from build123d import *

# Parameters (mm, degrees)
BOSS_EXTRUDE1_DEPTH                             = 76.2
BOSS_EXTRUDE1_DEPTH_BACK                        = 76.2
SKETCH3_W                                       = 76.2
SKETCH3_H                                       = 6.35
SKETCH11_R                                      = 13.97
CUT_EXTRUDE1_DEPTH                              = 86.430512699
CSK_FOR_M4_FLAT_HEAD_MACHINE_SCREW1_D           = 4.5
CSK_FOR_M4_FLAT_HEAD_MACHINE_SCREW1_CSINK_D     = 9.4
CSK_FOR_M4_FLAT_HEAD_MACHINE_SCREW1_CSINK_ANGLE = 90
SKETCH20_W                                      = 76.2
SKETCH20_H                                      = 76.2
CUT_EXTRUDE2_DEPTH                              = 86.430512699
M3X0_5_TAPPED_HOLE3_D                           = 2.5
M3X0_5_TAPPED_HOLE3_DEPTH                       = 11.948924226
M3X0_5_TAPPED_HOLE3_TIP                         = 0.751075774


with BuildPart() as part:
    # Sketch3 → Boss-Extrude1 (new, two sides: drawn at the far end of the back side and taken through both)
    with BuildSketch(Plane.XY.offset(-BOSS_EXTRUDE1_DEPTH_BACK)):
        Rectangle(SKETCH3_W, SKETCH3_H)
    extrude(amount=BOSS_EXTRUDE1_DEPTH + BOSS_EXTRUDE1_DEPTH_BACK)

    # Sketch11 → Cut-Extrude1 (cut, through all)
    with BuildSketch(Plane.XZ.offset(3.175)):
        with Locations(Location((-0.450951641, 31.810066373, 0), (0, 0, 270))):
            Circle(SKETCH11_R)
    extrude(amount=-CUT_EXTRUDE1_DEPTH, mode=Mode.SUBTRACT)

    # CSK for M4 Flat Head Machine Screw1 (through all)
    with Locations(Plane(origin=(0, -3.175, 0), x_dir=(-1, 0, 0), z_dir=(0, -1, 0))):
        with Locations((11.200951641, -13.190520192), (-21.049048359, -31.810066373), (11.200951641, -50.429612554)):
            CounterSinkHole(CSK_FOR_M4_FLAT_HEAD_MACHINE_SCREW1_D / 2, CSK_FOR_M4_FLAT_HEAD_MACHINE_SCREW1_CSINK_D / 2, counter_sink_angle=CSK_FOR_M4_FLAT_HEAD_MACHINE_SCREW1_CSINK_ANGLE)

    # Sketch20 → Cut-Extrude2 (cut, through all)
    with BuildSketch(Plane.XZ.offset(3.175)):
        with Locations((0, -38.1)):
            Rectangle(SKETCH20_W, SKETCH20_H)
    extrude(amount=-CUT_EXTRUDE2_DEPTH, mode=Mode.SUBTRACT)

    # M3x0.5 Tapped Hole3
    with Locations(Plane.XY.offset(76.2)):
        with Locations((19.05, 0), (-19.05, 0)):
            Hole(M3X0_5_TAPPED_HOLE3_D / 2, depth=M3X0_5_TAPPED_HOLE3_DEPTH)
            with Locations((0, 0, -(M3X0_5_TAPPED_HOLE3_DEPTH + M3X0_5_TAPPED_HOLE3_TIP / 2))):  # 118° drill point
                Cone(0, M3X0_5_TAPPED_HOLE3_D / 2, M3X0_5_TAPPED_HOLE3_TIP, mode=Mode.SUBTRACT)


solid = part.part
Work out the finished part from the listing and answer in its coordinate system (mm). A direction names the side the tool comes from. Give positions to 0.01 mm unless a question says otherwise; leave off trailing zeros. Order: outer loops, then holes, each group sorted by start corner. A loop starts at its lowest first (then second) coordinate and runs counter-clockwise, first axis right, second up. Notation, with made-up numbers: (-4.5, 54) -> (1.5, 54) arc R11 cw to (1.5, 61) -> close; hole circle Ø8 at (-7, -5.5). An arc over 180 degrees is marked (long way). Answer as a JSON object with one key per item and string values. Group by question number.
1. Section A-A on z = 22 is taken. Determine the outline of the cut face in (x, y) (3 decimals), plus the area to 3 significant figures.
2. A flat-ended cylindrical pin translates along its axis: pin 1 Ø2.5 at (x, z) = (-11.2, 13.19) entering from -Y. Find the tip coordinate at first contact, or state that the pin passes through.
3. The mould has two halves that part along Y. Classify faces 1 (the flat face through (-1, 3.175, 46)), 2 (the conical face through (-11.71, -0.84, 52.74)), 3 (the conical face through (-18.85, -0.08, 63.63)): released by +Y, released by -Y, zero draft, split by the parting line, or undercut.
4. Consider line 1 along X through (y, z) = (0, 68.5); line 2 along Z through (x, y) = (0, -2.5); line 3 along X through (y, z) = (2, 30.5). Determine where each line is inside the solid, lowest interval first. Write a range as [from, to].
5. Section B-B on x = -5 is taken. Determine the outline of the cut face in (y, z) (3 decimals).
6. A tool of negligible diameter and unlimited length cuts with its end or side. For faces 4 (the cylindrical face through (-17.8, 0.05, 70.14)), 5 (the conical face through (-11.71, -0.84, 15.5)), from which of +Z, -Z, +X, -X, +Y, -Y can it reach the whole face along a straight path? Write none if from no direction.
7. Section C-C on y = -2.25 is taken. Determine the outline of the cut face in (x, z) (3 decimals), plus the area to 3 significant figures.
Result sheet:
{
 "1": {"outline": "(-38.1, -3.175) -> (-10.397, -3.175) -> (-10.397, 3.175) -> (-38.1, 3.175) -> close; (9.495, -3.175) -> (38.1, -3.175) -> (38.1, 3.175) -> (9.495, 3.175) -> close", "area": "358 mm^2"},
 "2": {"pin 1": "passes through"},
 "3": {"face 1": "released by +Y", "face 2": "released by -Y", "face 3": "undercut"},
 "4": {"line 1": "x = [-38.1, -20.3], [-17.8, 17.8], [20.3, 38.1]", "line 2": "z = [0, 17.85], [45.77, 76.2]", "line 3": "x = [-38.1, -14.36], [13.46, 19.22], [22.88, 38.1]"},
 "5": {"outline": "(-3.175, 0) -> (3.175, 0) -> (3.175, 18.601) -> (-3.175, 18.601) -> close; (-3.175, 45.019) -> (3.175, 45.019) -> (3.175, 76.2) -> (-3.175, 76.2) -> close"},
 "6": {"face 4": "+Z", "face 5": "-Y"},
 "7": {"outline": "(-38.1, 0) -> (38.1, 0) -> (38.1, 76.2) -> (-38.1, 76.2) -> close; hole circle Ø7.55 at (-11.201, 13.191); hole circle Ø7.55 at (-11.201, 50.43); hole circle Ø27.94 at (-0.451, 31.81); hole circle Ø7.55 at (21.049, 31.81)", "area": "5,060 mm^2"}
}
